The figure shows three views and two pictorial views of one solid part (mm, origin at its lowest corner). Answer the questions. Give positions to 0.01 mm unless a question says otherwise; leave off trailing zeros. Write each loop counter-clockwise with the first axis right and the second up, starting at its lowest first coordinate (ties: lowest second). Pieces come first, ordered by that corner, then holes. Notation, with made-up numbers: (7.5, -40) -> (17.5, -40) arc R20 cw to (17.5, -21) -> close; hole circle Ø9 at (74, 53). An arc over 180 degrees is marked (long way). Answer as CSV lines item,"result". Start each with the question number.
1. Find the intervals of material crossed by line 1 (X direction, y = 46, z = 0.1); line 2 (X direction, y = 110, z = 1.05) (1 decimal); line 3 (Y direction, x = 25, z = 1.15) (1 decimal), in increasing order.
2. Given pin 1 (1 mm diameter, centred on y = 24, z = 1, fed in from -X); pin 2 (1 mm diameter, centred on x = 31, z = 1, fed in from +Y), each flat-ended and moving along its own axis, determine where each tip first touches the part or whether it passes through.
3. The part is cut by section B-B, the plane y = 84.5. Determine the outline of the cut face in (x, z) (1 decimal).
4. The part is cut by section A-A, the plane z = 0.65. Determine the outline of the cut face in (x, y), and give its area (3 significant figures).
5. The part is cut by section D-D, the plane y = 24.5. Determine the outline of the cut face in (x, z), and give its area (3 significant figures).
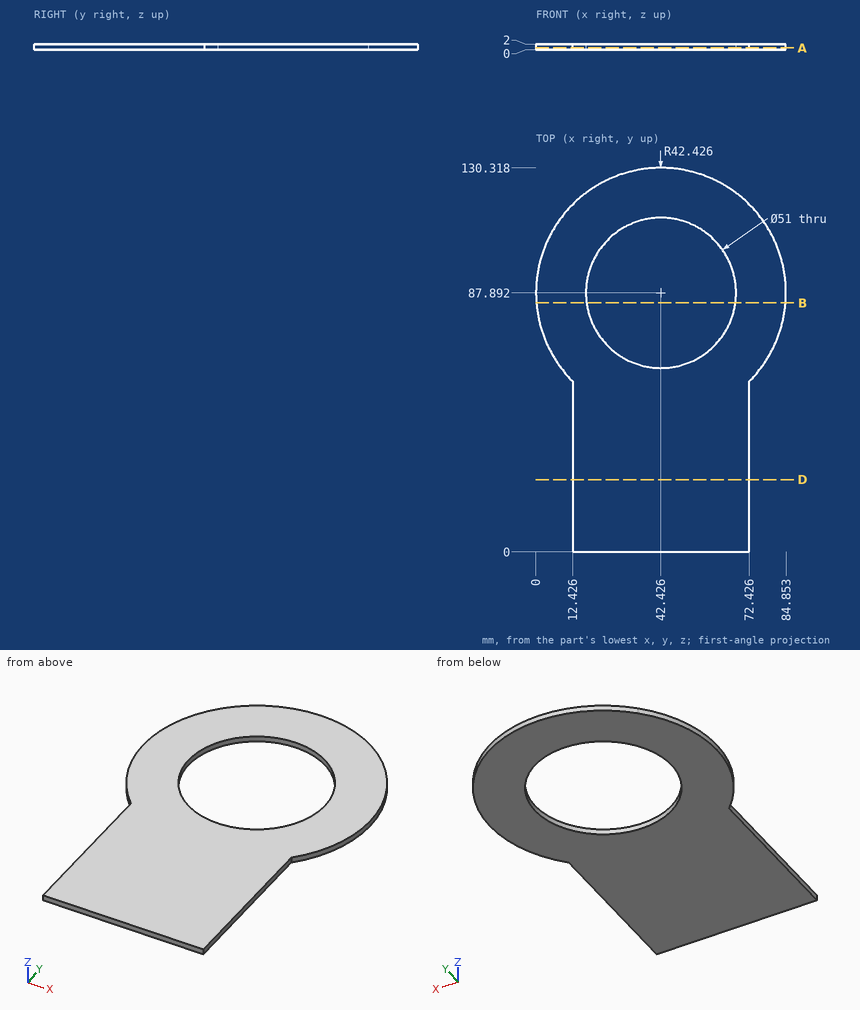
Results found:
1,line 1,"x = 12.43 to 72.43"
1,line 2,"x = 6.2 to 29.7, 55.1 to 78.6"
1,line 3,"y = 0 to 69.3, 106.5 to 126.6"
2,pin 1,"stops at x = 12.43"
2,pin 2,"stops at y = 128.89"
3,outline,"(0.1, 0) -> (17.2, 0) -> (17.2, 2) -> (0.1, 2) -> close; (67.7, 0) -> (84.7, 0) -> (84.7, 2) -> (67.7, 2) -> close"
4,outline,"(12.43, 0) -> (72.43, 0) -> (72.43, 57.89) arc R42.43 ccw (long way) to (12.43, 57.89) -> close; hole circle Ø51 at (42.43, 87.89)"
4,area,"6,570 mm²"
5,outline,"(12.43, 0) -> (72.43, 0) -> (72.43, 2) -> (12.43, 2) -> close"
5,area,"120 mm²"
